```python
from build123d import *

# Parameters (mm, degrees)
BASE_DEPTH                        = 6
SKETCH2_R                         = 1.5
SCREWS_CUT_DEPTH                  = 1
SCREWS_CUT_DEPTH_BACK             = 7
SKETCH4_W                         = 60.4
SKETCH4_H                         = 15.7
LCD_CUT_DEPTH                     = 1
LCD_CUT_DEPTH_BACK                = 7
SKETCH5_R                         = 3.75
TESTBUTTON_BIG_CUT_DEPTH          = 1
TESTBUTTON_BIG_CUT_DEPTH_BACK     = 7
SKETCH6_R                         = 4
SKETCH6_R_2                       = 3.25
TESTBUTTON_PIECE_MAINTAINER_DEPTH = 1
SKETCH7_R                         = 3.425
BRIGHTNESS_CUT_DEPTH              = 1
BRIGHTNESS_CUT_DEPTH_BACK         = 7
SKETCH8_R                         = 3.5
SKETCH8_R_2                       = 3
BRIGHTNESS_BACK_CUT_DEPTH         = 4


with BuildPart() as part:
    # Sketch1 → Base (new body)
    with BuildSketch(Plane.XY):
        with BuildLine():
            Line((-35.5, 19), (35.5, 19))
            ThreePointArc((35.5, 19), (36.964466094, 15.464466094), (40.5, 14))
            Line((40.5, 14), (40.5, -14))
            ThreePointArc((40.5, -14), (36.964466094, -15.464466094), (35.5, -19))
            Line((35.5, -19), (-35.5, -19))
            ThreePointArc((-35.5, -19), (-36.964466094, -15.464466094), (-40.5, -14))
            Line((-40.5, -14), (-40.5, 14))
            ThreePointArc((-40.5, 14), (-36.964466094, 15.464466094), (-35.5, 19))
        make_face()
    extrude(amount=BASE_DEPTH)

    # Sketch2 → Screws Cut (cut, two sides)
    with BuildSketch(Plane.XY.offset(6)) as screws_cut_sk:
        with Locations((-37.5, 0)):
            Circle(SKETCH2_R)
        with Locations((37.5, 0)):
            Circle(SKETCH2_R)
    extrude(amount=SCREWS_CUT_DEPTH, mode=Mode.SUBTRACT)
    extrude(screws_cut_sk.sketch, amount=-SCREWS_CUT_DEPTH_BACK, mode=Mode.SUBTRACT)

    # Sketch4 → LCD Cut (cut, two sides)
    with BuildSketch(Plane.XY.offset(6)) as lcd_cut_sk:
        with Locations((0, 7.85)):
            Rectangle(SKETCH4_W, SKETCH4_H)
    extrude(amount=LCD_CUT_DEPTH, mode=Mode.SUBTRACT)
    extrude(lcd_cut_sk.sketch, amount=-LCD_CUT_DEPTH_BACK, mode=Mode.SUBTRACT)

    # Sketch5 → TestButton Big Cut (cut, two sides)
    with BuildSketch(Plane.XY.offset(6)) as testbutton_big_cut_sk:
        with Locations((-27.5, -11.5)):
            Circle(SKETCH5_R)
    extrude(amount=TESTBUTTON_BIG_CUT_DEPTH, mode=Mode.SUBTRACT)
    extrude(testbutton_big_cut_sk.sketch, amount=-TESTBUTTON_BIG_CUT_DEPTH_BACK, mode=Mode.SUBTRACT)

    # Sketch6 → TestButton Piece Maintainer (add)
    with BuildSketch(Plane.XY.offset(6)):
        with Locations((-27.5, -11.5)):
            Circle(SKETCH6_R)
        with Locations((-27.5, -11.5)):
            Circle(SKETCH6_R_2, mode=Mode.SUBTRACT)
    extrude(amount=-TESTBUTTON_PIECE_MAINTAINER_DEPTH)

    # Sketch7 → Brightness Cut (cut, two sides)
    with BuildSketch(Plane.XY.offset(6)) as brightness_cut_sk:
        with Locations((25.5, -9)):
            Circle(SKETCH7_R)
    extrude(amount=BRIGHTNESS_CUT_DEPTH, mode=Mode.SUBTRACT)
    extrude(brightness_cut_sk.sketch, amount=-BRIGHTNESS_CUT_DEPTH_BACK, mode=Mode.SUBTRACT)

    # Sketch8 → Brightness Back Cut (add)
    with BuildSketch(Plane.XY.offset(6)):
        with Locations((25.5, -9)):
            Circle(SKETCH8_R)
        with Locations((25.5, -9)):
            Circle(SKETCH8_R_2, mode=Mode.SUBTRACT)
    extrude(amount=-BRIGHTNESS_BACK_CUT_DEPTH)


solid = part.part
```
Source: CAD feature listing. Evaluate the final solid. Frame: model axes, mm. A direction names the side the tool comes from. Round coordinates to 2 decimals unless told otherwise and drop trailing zeros. Write each loop counter-clockwise with the first axis right and the second up, starting at its lowest first coordinate (ties: lowest second). Pieces come first, ordered by that corner, then holes. Notation, with made-up numbers: M 72.5,10.25 L 89.5,10.25 A22 cw 89.5,47.25 Z; hole C 75.5,68.5 d6. An arc over 180 degrees is marked long. Answer as a JSON object with one key per item and string values. Group by question number.
(1) Reachability of faces 4 (the cylindrical face through (22.08, -8.85, 1.01)), 5 (the flat face through (30.2, 8, 3)), 6 (the flat face through (0, -19, 3)) from +Z, -Z, +X, -X, +Y, -Y: full face, straight path, thin tool, end or side. Return the list, or none.
(2) Section query A-A on y = 9.5. Output: boundary loops of the cut face in (x, z), then the cut area to 3 significant figures.
(3) Ray query, line 1 (Y direction, x = -27.5, z = 5.5); line 2 (X direction, y = 6.5, z = 2.1); line 3 (Y direction, x = -27.5, z = 1.4). Return the intervals inside material, ascending. Write a range as [from, to].
(4) Section query C-C on z = 3.35. Output: boundary loops of the cut face in (x, y), then the cut area to 3 significant figures.
(5) Section query B-B on x = -18. Output: boundary loops of the cut face in (y, z).
(6) Section query D-D on y = -10. Output: boundary loops of the cut face in (x, z), then the cut area to 3 significant figures.
(7) Mould query, pull axis Y, two halves, no side actions, for faces 1 (the flat face through (-30.2, 8, 3)), 2 (the cylindrical face through (-37, 15.43, 2.96)), 3 (the flat face through (40.5, 0, 3)). Classes: +Y half, -Y half, draft (parallel to the pull), parting line (faces both ways), or undercut.
Computed values:
{
 "1": {"face 4": "-Z", "face 5": "+Z, -Z", "face 6": "+Z, -Z, +X, -X, -Y"},
 "2": {"outline": "M -40.5,0 L -30.2,0 L -30.2,6 L -40.5,6 Z; M 30.2,0 L 40.5,0 L 40.5,6 L 30.2,6 Z", "area": "124 mm^2"},
 "3": {"line 1": "[-19, -14.75], [-8.25, 0], [15.7, 19]", "line 2": "[-40.5, -30.2], [30.2, 40.5]", "line 3": "[-19, -15.25], [-7.75, 0], [15.7, 19]"},
 "4": {"outline": "M -40.5,-14 A5 cw -35.5,-19 L 35.5,-19 A5 cw 40.5,-14 L 40.5,14 A5 cw 35.5,19 L -35.5,19 A5 cw -40.5,14 Z; hole C -37.5,0 d3; hole C -27.5,-11.5 d7.5; hole M -30.2,0 L 30.2,0 L 30.2,15.7 L -30.2,15.7 Z; hole C 25.5,-9 d6; hole C 37.5,0 d3", "area": "1,960 mm^2"},
 "5": {"outline": "M -19,0 L 0,0 L 0,6 L -19,6 Z; M 15.7,0 L 19,0 L 19,6 L 15.7,6 Z"},
 "6": {"outline": "M -40.5,0 L -30.94,0 L -30.94,5 L -30.38,5 L -30.38,6 L -40.5,6 Z; M -24.62,5 L -24.06,5 L -24.06,0 L 22.22,0 L 22.22,2 L 22.67,2 L 22.67,6 L -24.62,6 Z; M 28.33,2 L 28.78,2 L 28.78,0 L 40.5,0 L 40.5,6 L 28.33,6 Z", "area": "410 mm^2"},
 "7": {"face 1": "undercut", "face 2": "+Y half", "face 3": "draft"}
}
